The figure shows three views and two pictorial views of one solid part (mm, origin at its lowest corner). Answer the questions. Coordinates: 2 decimals unless noted, no trailing zeros. Write each loop counter-clockwise with the first axis right and the second up, starting at its lowest first coordinate (ties: lowest second). Pieces come first, ordered by that corner, then holes.
Item 1: Each of these flat-tipped pins is pushed along its axis until it touches: P1, Ø1.1, axis at x = 34.5, y = 1.5, coming from the -Z side; P2, Ø3, axis at x = 27.5, z = 10.5, coming from the -Y side; P3, Ø1.5, axis at x = 9, y = 2.5, coming from the +Z side. Where does it stop, or does it pass through?
Item 2: Section B-B (x = 25) is taken. Give the vertices of the cut face in (y, z), then the cut area to 3 significant figures.
Item 3: Straight lines are drawn through the part: probe 1 along X at (y, z) = (2.5, 34.5); probe 2 along Z at (x, y) = (26, 3.5); probe 3 along Y at (x, z) = (19.5, 35.5). For each, find the intervals that lie inside material, in ascending order.
Item 4: Determine the mould class of the marked faces 1 and 2 for opening direction Z: released by +Z, released by -Z, zero draft, split by the parting line, or undercut.
Item 5: Section C-C (z = 18.5) is taken. Give the vertices of the cut face in (x, y), then the cut area to 3 significant figures.
Item 6: Section A-A (y = 2.5) is taken. Give the vertices of the cut face in (x, z), then the cut area to 3 significant figures.
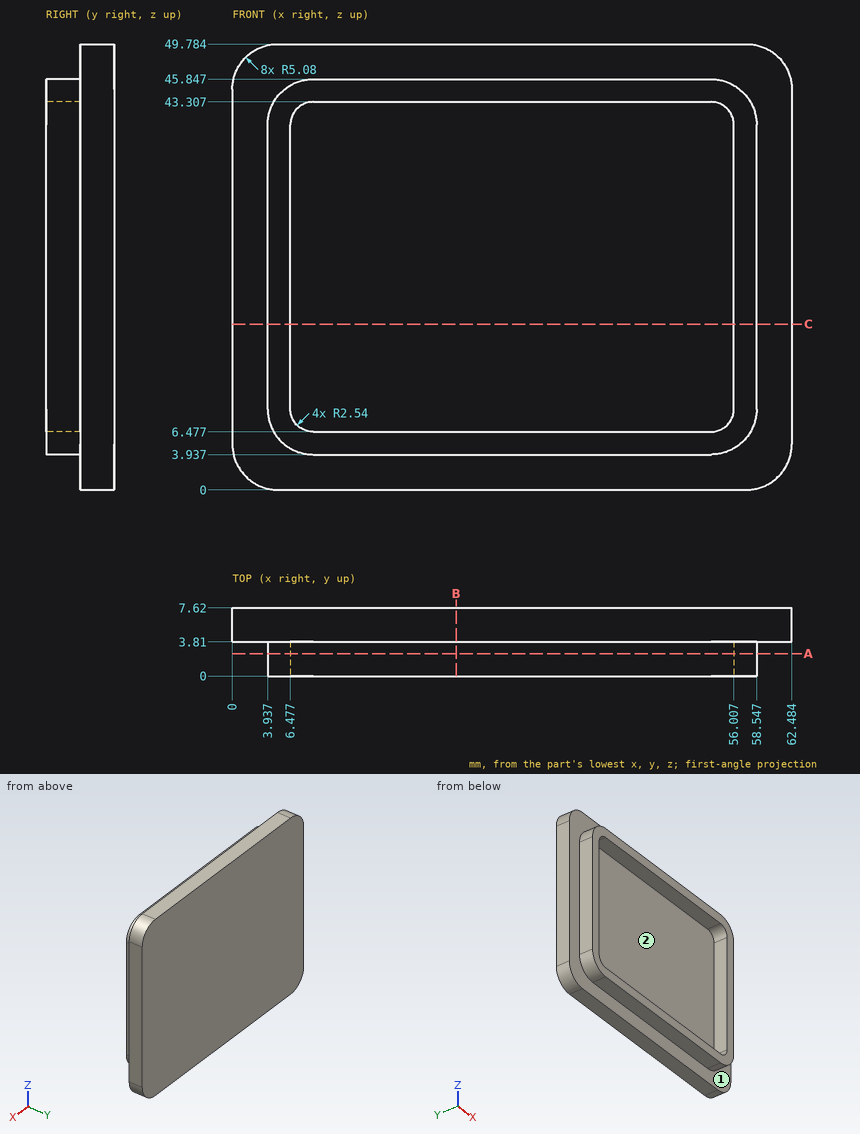
Established:
1. P1: stops at z = 3.94
1. P2: stops at y = 3.81
1. P3: stops at z = 45.85
2. outline: (0, 3.94) - (3.81, 3.94) - (3.81, 0) - (7.62, 0) - (7.62, 49.78) - (3.81, 49.78) - (3.81, 45.85) - (0, 45.85) - (0, 43.31) - (3.81, 43.31) - (3.81, 6.48) - (0, 6.48) - close
2. area: 209 mm2
3. probe 1: x = 3.94 to 6.48, 56.01 to 58.55
3. probe 2: z = 3.94 to 6.48, 43.31 to 45.85
3. probe 3: y = 3.81 to 7.62
4. face 1: zero draft
4. face 2: undercut
5. outline: (0, 3.81) - (3.94, 3.81) - (3.94, 0) - (6.48, 0) - (6.48, 3.81) - (56.01, 3.81) - (56.01, 0) - (58.55, 0) - (58.55, 3.81) - (62.48, 3.81) - (62.48, 7.62) - (0, 7.62) - close
5. area: 257 mm2
6. outline: (3.94, 9.02) arc R5.08 ccw to (9.02, 3.94) - (53.47, 3.94) arc R5.08 ccw to (58.55, 9.02) - (58.55, 40.77) arc R5.08 ccw to (53.47, 45.85) - (9.02, 45.85) arc R5.08 ccw to (3.94, 40.77) - close; hole (6.48, 9.02) arc R2.54 ccw to (9.02, 6.48) - (53.47, 6.48) arc R2.54 ccw to (56.01, 9.02) - (56.01, 40.77) arc R2.54 ccw to (53.47, 43.31) - (9.02, 43.31) arc R2.54 ccw to (6.48, 40.77) - close
6. area: 448 mm2
